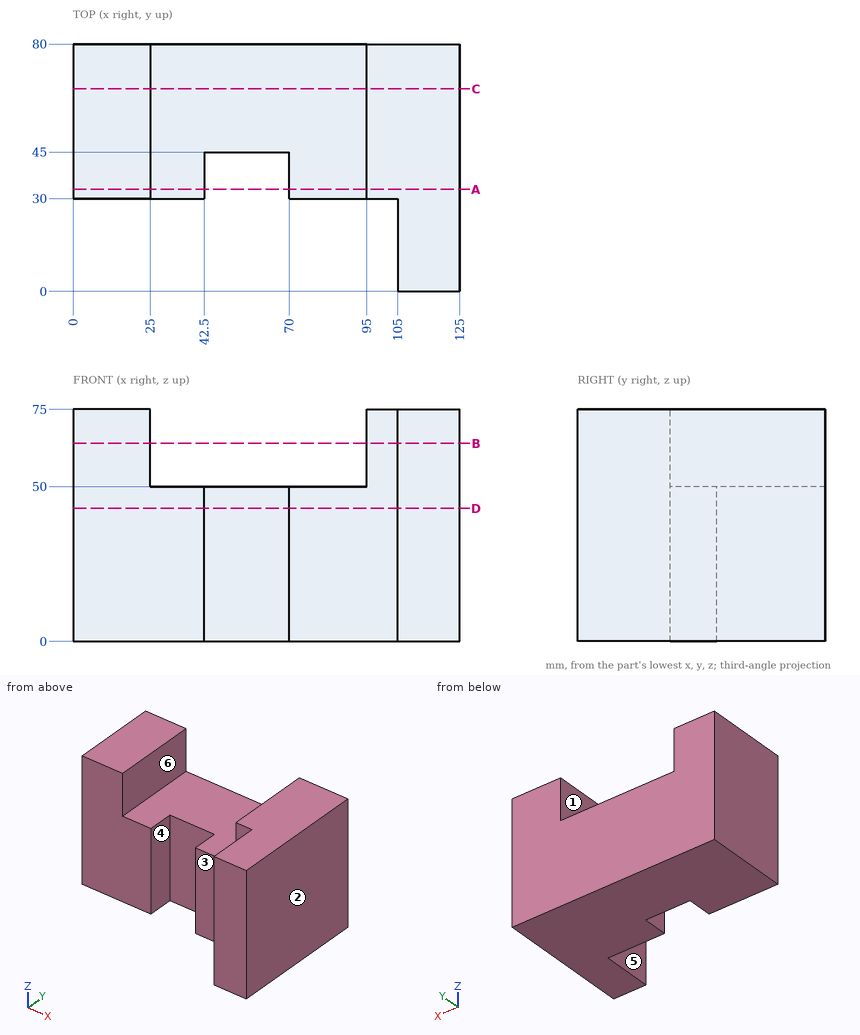
Job drawing, mm, ordinate dimensions from the low corner. One solid piece. A direction names the side the tool comes from. Give positions to 0.01 mm unless a question says otherwise; leave off trailing zeros. Loops run counter-clockwise (first coordinate to the right, second up) from the corner with the lowest first, then second, coordinate; pieces in that order, holes last.
Item 1: Slice it at A-A, the plane y = 33. List the corners of the cut face in (x, z).
Answers follow:
outline: (0, 0) - (42.5, 0) - (42.5, 50) - (25, 50) - (25, 75) - (0, 75) - close; (70, 0) - (125, 0) - (125, 75) - (95, 75) - (95, 50) - (70, 50) - close
Item 2: Which spindle directions (+Z, -Z, +X, -X, +Y, -Y) get a long thin tool onto all of the face, cutting with end or side? Do the marked faces 4, 5 and 6. Say none if no direction does.
Answers follow:
face 4: +Z, -Z, -Y
face 5: +Z, -Z, -X, -Y
face 6: +Z, +Y, -Y
Item 3: Pull direction X, two halves, no side cores. Call the marked faces 1, 2 and 3: released by +X, released by -X, zero draft, split by the parting line, or undercut.
Answers follow:
face 1: undercut
face 2: released by +X
face 3: zero draft
Item 4: Drill centre lines: line 1 (X direction, y = 50.5, z = 70); line 2 (Y direction, x = 104, z = 48); line 3 (Z direction, x = 80.5, y = 44). Where is each one in solid material? Low to high.
Answers follow:
line 1: x = 0 to 25, 95 to 125
line 2: y = 30 to 80
line 3: z = 0 to 50
Item 5: Slice it at C-C, the plane y = 65.5. List the corners of the cut face in (x, z).
Answers follow:
outline: (0, 0) - (125, 0) - (125, 75) - (95, 75) - (95, 50) - (25, 50) - (25, 75) - (0, 75) - close
Item 6: Flat gauge pins, fed straight in: pin 1 (2 mm diameter, centred on x = 78, z = 36, fed in from -Y); pin 2 (5 mm diameter, centred on x = 72, y = 36, fed in from +Z); pin 3 (24 mm diameter, centred on y = 9, z = 53.5, fed in from -X). Where does each tip first touch, or does it go through?
Answers follow:
pin 1: stops at y = 30
pin 2: stops at z = 50
pin 3: stops at x = 105
Item 7: Slice it at D-D, the plane z = 43. List the corners of the cut face in (x, y).
Answers follow:
outline: (0, 30) - (42.5, 30) - (42.5, 45) - (70, 45) - (70, 30) - (105, 30) - (105, 0) - (125, 0) - (125, 80) - (0, 80) - close
Item 8: Slice it at B-B, the plane z = 64. List the corners of the cut face in (x, y).
Answers follow:
outline: (0, 30) - (25, 30) - (25, 80) - (0, 80) - close; (95, 30) - (105, 30) - (105, 0) - (125, 0) - (125, 80) - (95, 80) - close
